The listing builds one solid part. Answer for the finished solid, in the listing's coordinates (mm). Round coordinates to 2 decimals unless told otherwise and drop trailing zeros. Loops run counter-clockwise (first coordinate to the right, second up) from the corner with the lowest first, then second, coordinate; pieces in that order, holes last. Notation, with made-up numbers: (78.25, -18) -> (103.25, -18) arc R12 cw to (103.25, 1) -> close; hole circle Ø2 at (23, -19). An arc over 180 degrees is marked (long way). Use a Markdown table: item, result. Add a question column.
Q1. Section A-A on y = 1 is taken. Give the vertices of the cut face in (x, z).
Q2. Section B-B on z = 49 is taken. Give the vertices of the cut face in (x, y), then the cut area to 3 significant figures.
Q3. Consider line 1 (Z direction, x = 4.75, y = 2); line 2 (Z direction, x = 2.5, y = 2.25); line 3 (X direction, y = -0.25, z = 222). Determine where each line is inside the solid, lowest interval first.
from build123d import *

# Parameters (mm, degrees)
ESQUISSE1_W                     = 10
ESQUISSE1_H                     = 10
BOSS_EXTRU_1_DEPTH              = 234
BOSS_EXTRU_1_DEPTH_BACK         = 2
ESQUISSE2_W                     = 2
ESQUISSE2_H                     = 10
ESQUISSE2_W_2                   = 5
ENL_V_MAT_EXTRU_1_DEPTH         = 11
ESQUISSE3_W                     = 10
ESQUISSE3_H                     = 2
ENL_V_MAT_EXTRU_2_DEPTH         = 11
TROU_TARAUD_M3X0_51_D           = 2.5
TROU_TARAUD_M3X0_51_CSINK_D     = 3.05
TROU_TARAUD_M3X0_51_CSINK_ANGLE = 90


with BuildPart() as part:
    # Esquisse1 → Boss.-Extru.1 (new body, two sides)
    with BuildSketch(Plane.XY) as boss_extru_1_sk:
        Rectangle(ESQUISSE1_W, ESQUISSE1_H)
    extrude(amount=BOSS_EXTRU_1_DEPTH)
    extrude(boss_extru_1_sk.sketch, amount=-BOSS_EXTRU_1_DEPTH_BACK)

    # Esquisse2 → Enl_v. mat.-Extru.1 (cut, through all)
    with BuildSketch(Plane(origin=(0, 5, 0), x_dir=(1, 0, 0), z_dir=(0, 1, 0))):
        with Locations((4, -122.2)):
            Rectangle(ESQUISSE2_W, ESQUISSE2_H)
        with Locations((4, -184.2)):
            Rectangle(ESQUISSE2_W, ESQUISSE2_H)
        with Locations((4, -21.2)):
            Rectangle(ESQUISSE2_W, ESQUISSE2_H)
        with Locations((2.5, -47.4)):
            Rectangle(ESQUISSE2_W_2, ESQUISSE2_H)
    extrude(amount=-ENL_V_MAT_EXTRU_1_DEPTH, mode=Mode.SUBTRACT)

    # Esquisse3 → Enl_v. mat.-Extru.2 (cut, through all)
    with BuildSketch(Plane.ZY.offset(5)):
        with Locations((153.2, 4)):
            Rectangle(ESQUISSE3_W, ESQUISSE3_H)
    extrude(amount=-ENL_V_MAT_EXTRU_2_DEPTH, mode=Mode.SUBTRACT)

    # Trou taraud_ M3x0.51 (through all)
    with Locations(Plane(origin=(0, 5, 0), x_dir=(1, 0, 0), z_dir=(0, 1, 0))):
        with Locations((0, -222), (0, -10)):
            CounterSinkHole(TROU_TARAUD_M3X0_51_D / 2, TROU_TARAUD_M3X0_51_CSINK_D / 2, counter_sink_angle=TROU_TARAUD_M3X0_51_CSINK_ANGLE)


solid = part.part
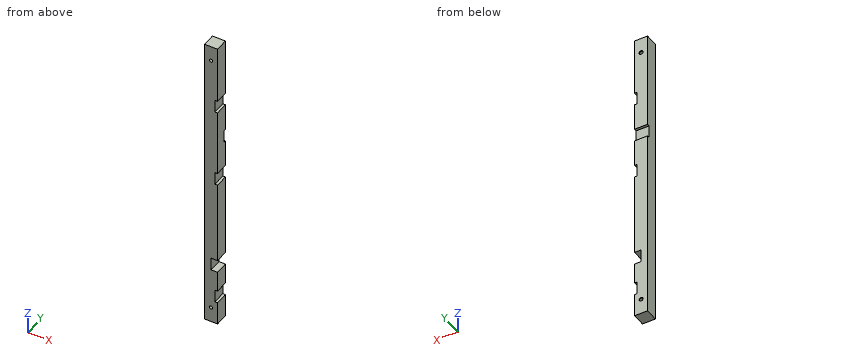
Checked values:
| question | item | result |
|---|---|---|
| 1 | outline | (-5, -2) -> (5, -2) -> (5, 16.2) -> (3, 16.2) -> (3, 26.2) -> (5, 26.2) -> (5, 42.4) -> (0, 42.4) -> (0, 52.4) -> (5, 52.4) -> (5, 117.2) -> (3, 117.2) -> (3, 127.2) -> (5, 127.2) -> (5, 179.2) -> (3, 179.2) -> (3, 189.2) -> (5, 189.2) -> (5, 234) -> (-5, 234) -> close; hole circle Ø2.5 at (0, 10); hole circle Ø2.5 at (0, 222) |
| 2 | outline | (-5, -5) -> (0, -5) -> (0, 5) -> (-5, 5) -> close |
| 2 | area | 50.0 mm2 |
| 3 | line 1 | z = -2 to 16.2, 26.2 to 42.4, 52.4 to 117.2, 127.2 to 179.2, 189.2 to 234 |
| 3 | line 2 | z = -2 to 42.4, 52.4 to 234 |
| 3 | line 3 | x = -5 to -1.25, 1.25 to 5 |
